Model file for the job. Use its own axes, mm. Give positions to 0.01 mm unless a question says otherwise; leave off trailing zeros. Write each loop counter-clockwise with the first axis right and the second up, starting at its lowest first coordinate (ties: lowest second). Pieces come first, ordered by that corner, then holes.
```python
from build123d import *

# Parameters (mm, degrees)
SKETCH1_R           = 10.5
SKETCH1_R_2         = 9.5
BOSS_EXTRUDE1_DEPTH = 263
BOSS_EXTRUDE2_DEPTH = 263
CUT_EXTRUDE1_DEPTH  = 264.564518904


with BuildPart() as part:
    # Sketch1 → Boss-Extrude1 (new body)
    # profile 1 of 3: a face of its own
    with BuildSketch(Plane.XY):
        with BuildLine():
            ThreePointArc((-10.5, 0), (-7.424621202, 7.424621202), (0, 10.5))
            Line((0, 10.5), (-10.5, 10.5))
            Line((-10.5, 10.5), (-10.5, 0))
        make_face()
    # profile 2 of 3: a face of its own
    with BuildSketch(Plane.XY):
        with BuildLine():
            Line((10.5, 10.5), (0, 10.5))
            ThreePointArc((0, 10.5), (7.424621202, 7.424621202), (10.5, 0))
            Line((10.5, 0), (10.5, 10.5))
        make_face()
    # profile 3 of 3: a face of its own
    with BuildSketch(Plane.XY):
        Circle(SKETCH1_R)
        Circle(SKETCH1_R_2, mode=Mode.SUBTRACT)
    extrude(amount=BOSS_EXTRUDE1_DEPTH)

    # Sketch2 → Boss-Extrude2 (add)
    with BuildSketch(Plane.XY.offset(263)):
        Polygon((-10.5, 13.675), (-10.5, 10.5), (-8.976, 10.5), (-8.976, 12.0748), (-8.976, 13.675), align=None)
        Polygon((-8.976, 13.675), (-8.976, 12.0748), (-7.3758, 12.0748), align=None)
        Polygon((7.4324, 12.086261455), (9.0326, 12.0875), (9.0326, 13.675), align=None)
        Polygon((9.0326, 12.0875), (9.0326, 10.5), (10.5, 10.5), (10.5, 13.675), (9.0326, 13.675), align=None)
    extrude(amount=-BOSS_EXTRUDE2_DEPTH)

    # Sketch3 → Cut-Extrude1 (cut, through all)
    with BuildSketch(Plane.XY.offset(263)):
        with BuildLine():
            ThreePointArc((-6.74608819, 6.688818591), (-5.154578199, 7.979995212), (-3.323185213, 8.8998))
            Line((-3.323185213, 8.8998), (-8.976, 8.8998))
            Line((-8.976, 8.8998), (-6.74608819, 6.688818591))
        make_face()
        with BuildLine():
            Line((3.323185213, 8.8998), (9.0326, 8.8998))
            Line((9.0326, 8.8998), (7.4324, 10.5))
            Line((7.4324, 10.5), (-7.3758, 10.5))
            Line((-7.3758, 10.5), (-8.976, 8.8998))
            Line((-8.976, 8.8998), (-3.323185213, 8.8998))
            ThreePointArc((-3.323185213, 8.8998), (0, 9.5), (3.323185213, 8.8998))
        make_face()
        with BuildLine():
            Line((6.767076018, 6.667584433), (9.0326, 8.8998))
            Line((9.0326, 8.8998), (3.323185213, 8.8998))
            ThreePointArc((3.323185213, 8.8998), (5.167111332, 7.971885629), (6.767076018, 6.667584433))
        make_face()
    extrude(amount=-CUT_EXTRUDE1_DEPTH, mode=Mode.SUBTRACT)


solid = part.part
```
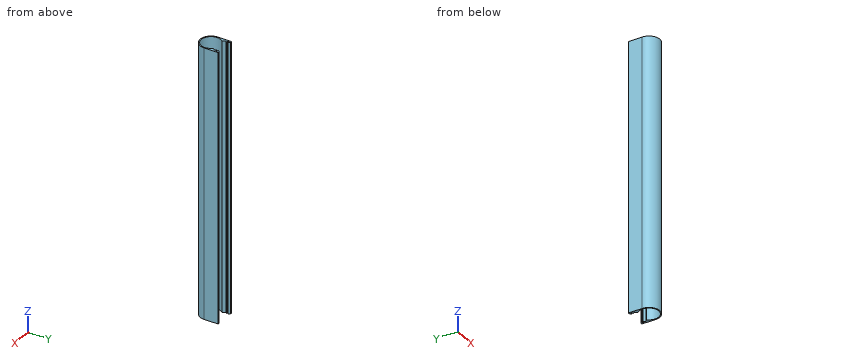
1. Probe probe 1 along X at (y, z) = (11.5, 215.5); probe 2 along Y at (x, z) = (7.75, 31); probe 3 along X at (y, z) = (-0.25, 111.5). List the from-to ranges inside material, lowest first.
Calculated:
probe 1: x = -10.5 to -8.98, 9.03 to 10.5
probe 2: y = -7.08 to -5.49, 5.49 to 7.64, 10.18 to 10.5, 12.09 to 12.4
probe 3: x = -10.5 to -9.5, 9.5 to 10.5
2. Slice it at A-A, the plane z = 180.5. Write the cut outline in (x, y) (1 decimal).
Calculated:
outline: (-10.5, 0) arc R10.5 ccw to (10.5, 0) - (10.5, 13.7) - (9, 13.7) - (7.4, 12.1) - (9, 12.1) - (9, 10.5) - (7.4, 10.5) - (9, 8.9) - (6.8, 6.7) arc R9.5 cw (long way) to (-6.7, 6.7) - (-9, 8.9) - (-7.4, 10.5) - (-9, 10.5) - (-9, 12.1) - (-7.4, 12.1) - (-9, 13.7) - (-10.5, 13.7) - close
3. Slice it at C-C, the plane x = 0. Write the cut outline in (y, z), and give its area (3 significant figures).
Calculated:
outline: (-10.5, 0) - (-9.5, 0) - (-9.5, 263) - (-10.5, 263) - close
area: 263 mm2
4. Pin check, flat tips, straight feed: P1, Ø2, axis at x = 4.5, z = 79, coming from the +Y side; P2, Ø0.5, axis at x = -8, z = 162, coming from the -Y side; P3, Ø1, axis at x = -1, z = 137, coming from the -Y side; P4, Ø12, axis at x = -8.5, z = 48.5, coming from the +Y side (3 decimals). Stop position of each tip, or through.
Calculated:
P1: stops at y = -7.75
P2: stops at y = -7.08
P3: stops at y = -10.49
P4: stops at y = 13.675
5. Slice it at B-B, the plane y = -6.5. Write the cut outline in (x, z), and give its area (3 significant figures).
Calculated:
outline: (-8.25, 0) - (-6.93, 0) - (-6.93, 263) - (-8.25, 263) - close; (6.93, 0) - (8.25, 0) - (8.25, 263) - (6.93, 263) - close
area: 693 mm2
